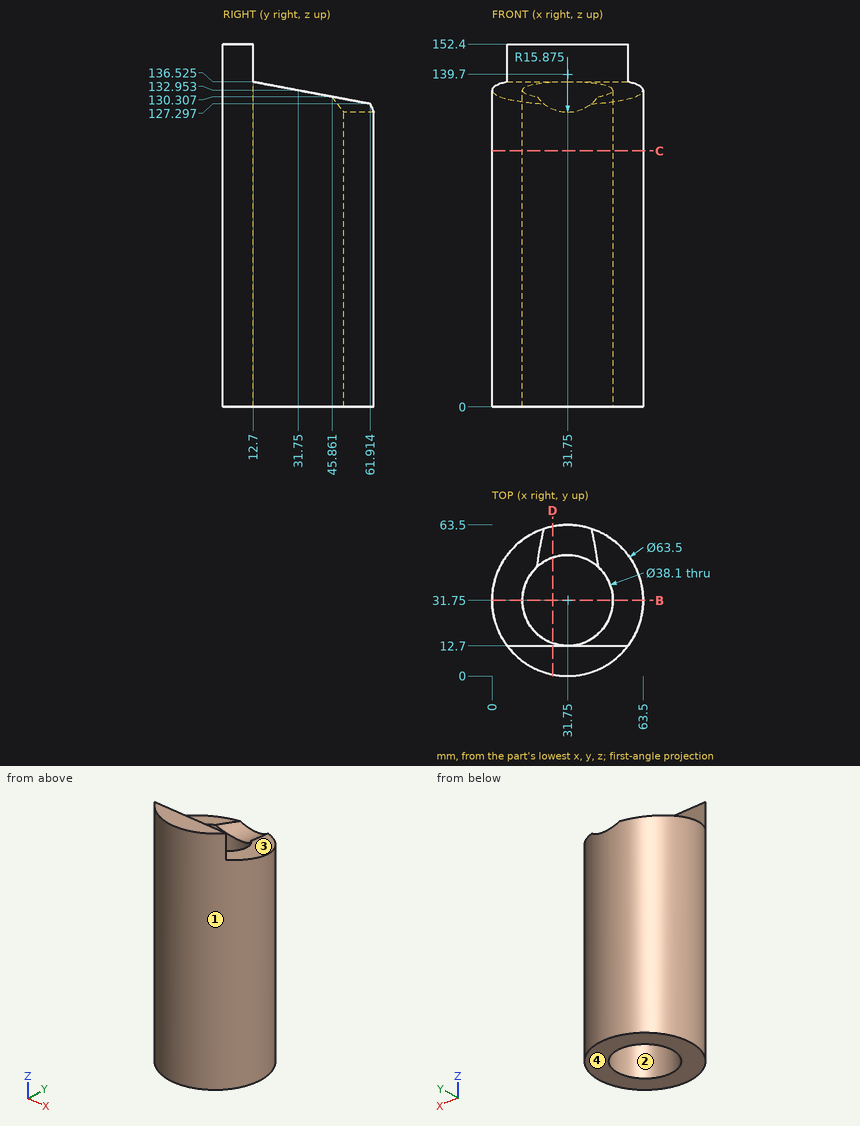
Study the drawing (mm; zero at the part's minimum x, y, z) and answer. Give positions to 0.01 mm unless a question says otherwise; leave off trailing zeros. Write each loop counter-clockwise with the first axis right and the second up, starting at its lowest first coordinate (ties: lowest second). Pieces come first, ordered by that corner, then holes. Notation, with made-up numbers: (25.5, 53) - (40.5, 53) arc R20 ccw to (40.5, 75) - close; hole circle Ø8 at (-22.5, 63.25). An arc over 180 degrees is marked (long way). One line per question, with ' | ' between items. Start each with the question number.
1. Given P1, Ø1.5, axis at y = 53, z = 77, coming from the -X side (1 decimal); P2, Ø8, axis at y = 11, z = 25.5, coming from the +X side; P3, Ø1.5, axis at y = 45, z = 121.5, coming from the +X side (1 decimal), each flat-ended and moving along its own axis, determine where each tip first touches the part or whether it passes through.
2. Section C-C, the plane z = 107.5 is taken. Determine the outline of the cut face in (x, y).
3. Straight lines are drawn through the part: line 1 (Y direction, x = 31.75, z = 49); line 2 (Y direction, x = 47.5, z = 72.5) (1 decimal). For each, find the intervals that lie inside material, in ascending order.
4. Section B-B, the plane y = 31.75 is taken. Determine the outline of the cut face in (x, z), then the cut area to 3 significant figures.
5. Determine the mould class of the marked faces 1, 2, 3 and 4 for opening direction Y: +Y half, -Y half, draft (parallel to the pull), parting line (faces both ways), or undercut.
6. Section D-D, the plane x = 25.5 is taken. Determine the outline of the cut face in (y, z) (1 decimal), then the cut area to 3 significant figures.
Result:
1) P1: stops at x = 7.5 | P2: stops at x = 58.72 | P3: stops at x = 60.9
2) outline: circle Ø63.5 at (31.75, 31.75); hole circle Ø38.1 at (31.75, 31.75)
3) line 1: y = 0 to 12.7, 50.8 to 63.5 | line 2: y = 4.2 to 21, 42.5 to 59.3
4) outline: (0, 0) - (12.7, 0) - (12.7, 132.95) - (0, 132.95) - close; (50.8, 0) - (63.5, 0) - (63.5, 132.95) - (50.8, 132.95) - close | area: 3,380 mm2
5) face 1: parting line | face 2: undercut | face 3: +Y half | face 4: draft
6) outline: (0.6, 0) - (13.8, 0) - (13.8, 136.3) - (12.7, 136.5) - (12.7, 152.4) - (0.6, 152.4) - close; (49.7, 0) - (62.9, 0) - (62.9, 125.1) - (49.7, 125.1) - close | area: 3,630 mm2
